Check sheet for the modelled part. Datum: model origin and axes. Units: mm. Face numbers are marked on the shaded views. A direction names the side the tool comes from. Coordinates: 2 decimals unless noted, no trailing zeros. Write each loop counter-clockwise with the first axis right and the second up, starting at its lowest first coordinate (ties: lowest second). Pieces come first, ordered by that corner, then holes. Notation, with made-up numbers: (81.25, 59.25) - (92.25, 59.25) arc R3 ccw to (92.25, 63.25) - close; hole circle Ø8 at (-40, 27.5). An arc over 180 degrees is marked (long way). Write each question's results on one line, items separated by ' | '.
from build123d import *

# Parameters (mm, degrees)
RESSALTO_EXTRUS_O1_DEPTH = 35
RESSALTO_EXTRUS_O1_TAPER = 15
ESBO_O2_W                = 39.326456566
ESBO_O2_H                = 52.605122422
CORTE_EXTRUS_O1_DEPTH    = 50
ESBO_O5_W                = 2.8
ESBO_O5_H                = 2.8
CORTE_EXTRUS_O2_DEPTH    = 97.382052271
CORTE_EXTRUS_O3_START    = -5
ESBO_O6_R                = 3
CORTE_EXTRUS_O3_DEPTH    = 20
CORTE_EXTRUS_O4_DEPTH    = 35
CORTE_EXTRUS_O4_DRAFT    = -15


with BuildPart() as part:
    # Esboço1 → Ressalto-extrusão1 (new body)
    with BuildSketch(Plane.XY):
        Polygon((63.5, -26.302561211), (63.5, 26.302561211), (26.302561211, 63.5), (-26.302561211, 63.5), (-63.5, 26.302561211), (-63.5, -26.302561211), (-26.302561211, -63.5), (26.302561211, -63.5), align=None)
    extrude(amount=RESSALTO_EXTRUS_O1_DEPTH, taper=RESSALTO_EXTRUS_O1_TAPER)

    # Esboço2 → Corte-extrusão1 (cut)
    with BuildSketch(Plane.XY):
        with Locations((43.836771717, 0)):
            Rectangle(ESBO_O2_W, ESBO_O2_H)
    extrude(amount=CORTE_EXTRUS_O1_DEPTH, mode=Mode.SUBTRACT)

    # Esboço5 → Corte-extrusão2 (cut, through all)
    with BuildSketch(Plane(origin=(0, 0, 0), x_dir=(-1, 0, 0), z_dir=(0, 0, -1))):
        with Locations((-16, 59.5)):
            Rectangle(ESBO_O5_W, ESBO_O5_H)
        Polygon((30.759144982, 55.366460967), (32.739043969, 53.38656198), (30.759144982, 51.406662992), (28.779245994, 53.38656198), align=None)
        with Locations((16, 59.5)):
            Rectangle(ESBO_O5_W, ESBO_O5_H)
        Polygon((53.38656198, 32.739043969), (55.366460967, 30.759144982), (53.38656198, 28.779245994), (51.406662992, 30.759144982), align=None)
        with Locations((59.5, 16)):
            Rectangle(ESBO_O5_W, ESBO_O5_H)
        with Locations((59.5, -16)):
            Rectangle(ESBO_O5_W, ESBO_O5_H)
        Polygon((55.366460967, -30.759144982), (53.38656198, -32.739043969), (51.406662992, -30.759144982), (53.38656198, -28.779245994), align=None)
        Polygon((32.739043969, -53.38656198), (30.759144982, -55.366460967), (28.779245994, -53.38656198), (30.759144982, -51.406662992), align=None)
        with Locations((16, -59.5)):
            Rectangle(ESBO_O5_W, ESBO_O5_H)
        with Locations((-16, -59.5)):
            Rectangle(ESBO_O5_W, ESBO_O5_H)
        Polygon((-30.759144982, -55.366460967), (-32.739043969, -53.38656198), (-30.759144982, -51.406662992), (-28.779245994, -53.38656198), align=None)
        Polygon((-53.38656198, -32.739043969), (-55.366460967, -30.759144982), (-53.38656198, -28.779245994), (-51.406662992, -30.759144982), align=None)
        with Locations((-59.5, -16)):
            Rectangle(ESBO_O5_W, ESBO_O5_H)
        with Locations((-59.5, 16)):
            Rectangle(ESBO_O5_W, ESBO_O5_H)
        Polygon((-55.366460967, 30.759144982), (-53.38656198, 32.739043969), (-51.406662992, 30.759144982), (-53.38656198, 28.779245994), align=None)
        Polygon((-32.739043969, 53.38656198), (-30.759144982, 55.366460967), (-28.779245994, 53.38656198), (-30.759144982, 51.406662992), align=None)
    extrude(amount=-CORTE_EXTRUS_O2_DEPTH, mode=Mode.SUBTRACT)

    # Esboço6 → Corte-extrusão3 (cut)
    with BuildSketch(Plane(origin=(0, 0, 0), x_dir=(-1, 0, 0), z_dir=(0, 0, -1)).offset(CORTE_EXTRUS_O3_START)):
        with Locations((-16, 59.5)):
            Circle(ESBO_O6_R)
        with Locations((16, 59.5)):
            Circle(ESBO_O6_R)
        with Locations((30.759144982, 53.38656198)):
            Circle(ESBO_O6_R)
        with Locations((53.38656198, 30.759144982)):
            Circle(ESBO_O6_R)
        with Locations((59.5, 16)):
            Circle(ESBO_O6_R)
        with Locations((59.5, -16)):
            Circle(ESBO_O6_R)
        with Locations((53.38656198, -30.759144982)):
            Circle(ESBO_O6_R)
        with Locations((30.759144982, -53.38656198)):
            Circle(ESBO_O6_R)
        with Locations((16, -59.5)):
            Circle(ESBO_O6_R)
        with Locations((-16, -59.5)):
            Circle(ESBO_O6_R)
        with Locations((-30.759144982, -53.38656198)):
            Circle(ESBO_O6_R)
        with Locations((-53.38656198, -30.759144982)):
            Circle(ESBO_O6_R)
        with Locations((-59.5, -16)):
            Circle(ESBO_O6_R)
        with Locations((-59.5, 16)):
            Circle(ESBO_O6_R)
        with Locations((-53.38656198, 30.759144982)):
            Circle(ESBO_O6_R)
        with Locations((-30.759144982, 53.38656198)):
            Circle(ESBO_O6_R)
    extrude(amount=-CORTE_EXTRUS_O3_DEPTH, mode=Mode.SUBTRACT)


with BuildPart() as corte_extrus_o4_tool:
    # Esboço9 → Corte-extrusão4 (with draft: the straight prism first)
    with BuildSketch(Plane(origin=(0, 0, 0), x_dir=(-1, 0, 0), z_dir=(0, 0, -1))):
        Polygon((22.988852712, 55.5), (-22.988852712, 55.5), (-55.5, 22.988852712), (-55.5, -22.988852712), (-22.988852712, -55.5), (22.988852712, -55.5), (55.5, -22.988852712), (55.5, 22.988852712), align=None)
    extrude(amount=-CORTE_EXTRUS_O4_DEPTH)
    # Corte-extrusão4: the draft: its side faces are tilted about the plane it starts from
    corte_extrus_o4_sides = [corte_extrus_o4_tool.faces().sort_by_distance(p)[0] for p in [
        (0, 55.5, 17.5),
        (39.244426356, 39.244426356, 17.5),
        (55.5, 0, 17.5),
        (39.244426356, -39.244426356, 17.5),
        (0, -55.5, 17.5),
        (-39.244426356, -39.244426356, 17.5),
        (-55.5, 0, 17.5),
        (-39.244426356, 39.244426356, 17.5),
    ]]
    draft(corte_extrus_o4_sides, Plane(origin=(0, 0, 0), x_dir=(-1, 0, 0), z_dir=(0, 0, -1)), CORTE_EXTRUS_O4_DRAFT)


with BuildPart() as part_1:
    add(part.part)

    # Corte-extrusão4: cut by corte_extrus_o4_tool
    add(corte_extrus_o4_tool.part, mode=Mode.SUBTRACT)


solid = part_1.part
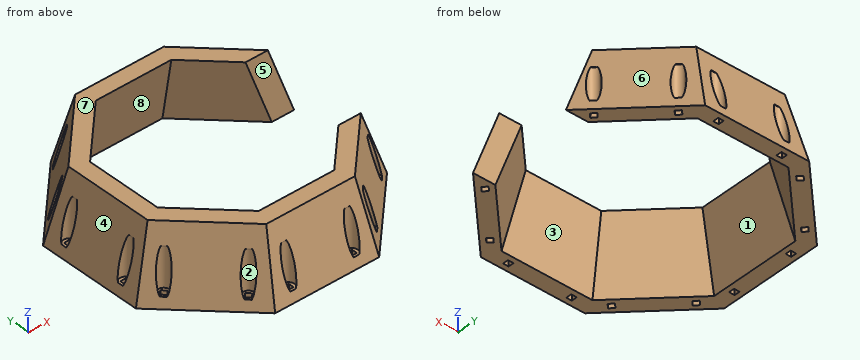
1. Sectioned sample at A-A (x = -8). Record the cut outline in (y, z).
Values follow:
outline: (-63.5, 0) - (-55.5, 0) - (-46.12, 35) - (-54.12, 35) - close; (46.12, 35) - (55.5, 0) - (63.5, 0) - (54.12, 35) - close
2. Go/stop test with flat-tipped pins: pin 1 (3.5 mm diameter, centred on x = -16, y = -59.5, fed in from -Z); pin 2 (2 mm diameter, centred on y = 59, z = 2.5, fed in from -X); pin 3 (5 mm diameter, centred on x = 16, y = -59.5, fed in from +Z); pin 4 (0.8 mm diameter, centred on y = 15.5, z = 3, fed in from -X). Record where each tip stops, or that it passes through.
Values follow:
pin 1: stops at z = 0 | pin 2: stops at x = -30.92 | pin 3: stops at z = 5 | pin 4: stops at x = -62.8
3. Material ranges on L1, parallel to X at y = -58, z = 16; L2, parallel to Y at x = -10.5, z = 20; L3, parallel to Y at x = 21, z = 25, recorded low to high. Write a range as [from, to].
Values follow:
L1: x = [-25.74, -18.6], [-13.4, 13.4], [18.6, 25.74] | L2: y = [-58.14, -50.14], [50.14, 58.14] | L3: y = [-56.8, -48.02], [48.02, 56.8]
4. Draft check along X on the marked faces 6, 7 and 8. Enter one of: pulls with the +X half, pulls with the -X half, needs draft (parallel to the pull), parting line crosses it, or undercut.
Values follow:
face 6: pulls with the +X half | face 7: needs draft | face 8: undercut
5. Access from +Z, -Z, +X, -X, +Y, -Y to the whole of each face (thin tool, end or side, straight path). Record for the marked faces 1, 2, 3, 4 and 5.
Values follow:
face 1: -Z, +X | face 2: none | face 3: -Z | face 4: +Z, -X, +Y, -Y | face 5: +Z, -Z, +X
6. Sectioned sample at B-B (z = 29.5). Record the cut outline in (x, y), then the cut area to 3 significant figures.
Values follow:
outline: (-55.6, -23.03) - (-23.03, -55.6) - (23.03, -55.6) - (52.32, -26.3) - (41.01, -26.3) - (19.71, -47.6) - (-19.71, -47.6) - (-47.6, -19.71) - (-47.6, 19.71) - (-19.71, 47.6) - (19.71, 47.6) - (41.01, 26.3) - (52.32, 26.3) - (23.03, 55.6) - (-23.03, 55.6) - (-55.6, 23.03) - close | area: 2,280 mm^2
